Input: part model. Units: mm. Frame: model coordinates. Face numbers are marked on the shaded views. A direction names the side the tool comes from. Give positions to 0.01 mm unless a question says otherwise; leave off trailing zeros. Write each loop counter-clockwise with the first axis right and the second up, starting at its lowest first coordinate (ties: lowest second). Pieces come first, ordered by that corner, then holes. Notation, with made-up numbers: (-20, 84) - (-12, 84) arc R26 cw to (-12, 120) - close; hole circle Ø1 at (21, -4). An arc over 180 degrees is marked (long way). Answer as CSV lines item,"result".
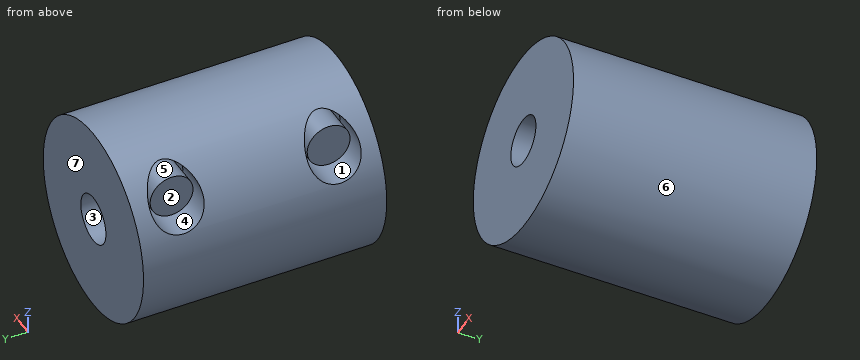
```python
from build123d import *

# Parameters (mm, degrees)
SKETCH1_R           = 10
SKETCH1_R_2         = 2.5
BOSS_EXTRUDE1_DEPTH = 25
CUT_EXTRUDE1_START  = -4
SKETCH2_R           = 2.702701275
CUT_EXTRUDE1_DEPTH  = 25.722813233
SKETCH3_R           = 2.202701275
BOSS_EXTRUDE2_DEPTH = 3


with BuildPart() as part:
    # Sketch1 → Boss-Extrude1 (new body)
    with BuildSketch(Plane(origin=(0, 0, 0), x_dir=(1, 0, 0), z_dir=(0, 1, 0))):
        with Locations(Location((0, 0, 0), (0, 0, 270))):
            Circle(SKETCH1_R)
        with Locations(Location((0, 0, 0), (0, 0, 270))):
            Circle(SKETCH1_R_2, mode=Mode.SUBTRACT)
    extrude(amount=BOSS_EXTRUDE1_DEPTH)

    # Sketch2 → Cut-Extrude1 (cut, through all)
    with BuildSketch(Plane(origin=(0, 0, 0), x_dir=(0, 0, -1), z_dir=(1, 0, 0)).offset(CUT_EXTRUDE1_START)):
        with Locations((-6.078771431, 20.570801258)):
            Circle(SKETCH2_R)
        with Locations((-6.078771431, 4.429198742)):
            Circle(SKETCH2_R)
    extrude(amount=-CUT_EXTRUDE1_DEPTH, mode=Mode.SUBTRACT)

    # Sketch3 → Boss-Extrude2 (add)
    with BuildSketch(Plane.ZY.offset(4)):
        with Locations((6.078771431, 4.429198742)):
            Circle(SKETCH3_R)
        with Locations(Location((6.078771431, 20.570801258, 0), (0, 0, 180))):
            Circle(SKETCH3_R)
    extrude(amount=BOSS_EXTRUDE2_DEPTH)


solid = part.part
```
Item 1: Ray query, line 1 (Y direction, x = -7.25, z = 5.75); line 2 (Y direction, x = -4.75, z = 8); line 3 (X direction, y = 16, z = 1). Return the intervals inside material, ascending. Write a range as from..to.
The answers:
line 1,"0..1.75, 7.11..17.89, 23.25..25"
line 2,"0..2.53, 3.35..5.51, 6.33..18.67, 19.49..21.65, 22.47..25"
line 3,"-9.95..-2.29, 2.29..9.95"
Item 2: Cut plane D-D on y = 10. Return the cut outline in (x, z), plus the area to 3 significant figures.
The answers:
outline,"circle Ø20 at (0, 0); hole circle Ø5 at (0, 0)"
area,"295 mm²"
Item 3: Contact query for flat-ended pins moving along their axis: pin 1 (5 mm diameter, centred on y = 20.5, z = 6, fed in from -X); pin 2 (2 mm diameter, centred on y = 14.5, z = -6, fed in from +X); pin 3 (2 mm diameter, centred on x = 4, y = 3, fed in from +Z). Output: stop coordinate, or through.
The answers:
pin 1,"x = -7"
pin 2,"x = 8.66"
pin 3,"z = 9.54"
Item 4: Mould query, pull axis Z, two halves, no side actions, for the marked faces 4, 5, 6 and 7. Classes: +Z half, -Z half, draft (parallel to the pull), parting line (faces both ways), or undercut.
The answers:
face 4,"undercut"
face 5,"undercut"
face 6,"parting line"
face 7,"draft"
Item 5: Cut plane A-A on z = 0. Return the cut outline in (x, y), plus the area to 3 significant figures.
The answers:
outline,"(-10, 0) - (-2.5, 0) - (-2.5, 25) - (-10, 25) - close; (2.5, 0) - (10, 0) - (10, 25) - (2.5, 25) - close"
area,"375 mm²"
Item 6: Cut plane C-C on x = 0. Return the cut outline in (y, z), plus the area to 3 significant figures.
The answers:
outline,"(0, -10) - (25, -10) - (25, -2.5) - (0, -2.5) - close; (0, 2.5) - (25, 2.5) - (25, 10) - (0, 10) - close"
area,"375 mm²"
Item 7: Reachability of the marked faces 1, 2 and 3 from +Z, -Z, +X, -X, +Y, -Y: full face, straight path, thin tool, end or side. Return the list, or none.
The answers:
face 1,"-X"
face 2,"+Z, -X"
face 3,"+Y, -Y"
Item 8: Cut plane B-B on x = -4.5. Return the cut outline in (y, z), plus the area to 3 significant figures.
The answers:
outline,"(0, -8.93) - (25, -8.93) - (25, 8.93) - (0, 8.93) - close; circle Ø4.41 at (4.43, 6.08); circle Ø4.41 at (20.57, 6.08); hole circle Ø5.41 at (4.43, 6.08); hole circle Ø5.41 at (20.57, 6.08)"
area,"431 mm²"
